Part print with two shaded views. Sizes in mm from the minimum x, y, z corner. Give positions to 0.01 mm unless a question says otherwise; leave off trailing zeros. Write each loop counter-clockwise with the first axis right and the second up, starting at its lowest first coordinate (ties: lowest second). Pieces come first, ordered by that corner, then holes. Notation, with made-up numbers: M 8.5,9.5 L 24.5,9.5 A27 cw 24.5,41.5 Z; hole C 57,-10 d6. An arc over 180 degrees is marked long. One line per item, written item: value. Start each with the question number.
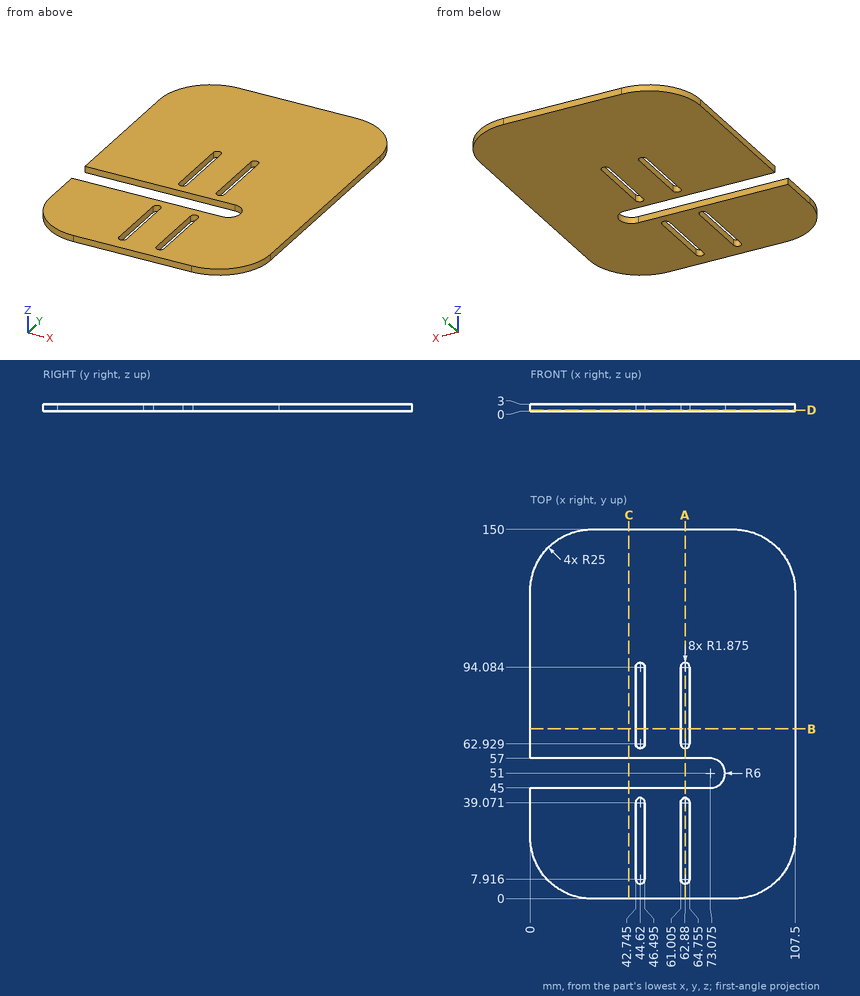
1) Band-saw the part on B-B (y = 69). List the corners of the cut face in (x, z) (1 decimal), then the cut area to 3 significant figures.
2) Band-saw the part on A-A (x = 62.88). List the corners of the cut face in (y, z).
3) Band-saw the part on C-C (x = 40). List the corners of the cut face in (y, z).
4) Probe line 1 along X through (y, z) = (87.5, 2.6) (1 decimal); line 2 along Y through (x, z) = (35, 2.1); line 3 along X through (y, z) = (16, 2.75) (1 decimal). List the from-to ranges inside material, lowest first. Write a range as from..to.
5) Drop flat-ended pins along their axis: P1, Ø0.9, axis at y = 23, z = 1.5, coming from the +X side; P2, Ø1.5, axis at x = 21, z = 2, coming from the +Y side; P3, Ø1.5, axis at y = 18, z = 2, coming from the -X side. Give the stop position or say it passes through.
6) Band-saw the part on D-D (z = 0.5). Count the separate pieces of the cut face and the enclosed holes in it, then the cut area to 3 significant figures.
Model answer:
1. outline: M 0,0 L 42.7,0 L 42.7,3 L 0,3 Z; M 46.5,0 L 61,0 L 61,3 L 46.5,3 Z; M 64.8,0 L 107.5,0 L 107.5,3 L 64.8,3 Z
1. area: 300 mm²
2. outline: M 0,0 L 6.04,0 L 6.04,3 L 0,3 Z; M 40.95,0 L 45,0 L 45,3 L 40.95,3 Z; M 57,0 L 61.05,0 L 61.05,3 L 57,3 Z; M 95.96,0 L 150,0 L 150,3 L 95.96,3 Z
3. outline: M 0,0 L 45,0 L 45,3 L 0,3 Z; M 57,0 L 150,0 L 150,3 L 57,3 Z
4. line 1: x = 0..42.7, 46.5..61, 64.8..107.5
4. line 2: y = 0..45, 57..150
4. line 3: x = 1.7..42.7, 46.5..61, 64.8..105.8
5. P1: stops at x = 107.45
5. P2: stops at y = 149.79
5. P3: stops at x = 0.79
6. separate pieces: 1
6. enclosed holes: 4
6. area: 14,100 mm²
